Geometry: final body of the model. Coordinates: model frame, mm. A direction names the side the tool comes from. Coordinates: 2 decimals unless noted, no trailing zeros. Write each loop counter-clockwise with the first axis right and the second up, starting at its lowest first coordinate (ties: lowest second). Pieces come first, ordered by that corner, then holes.
from build123d import *

# Parameters (mm, degrees)
SKETCH_1_R      = 1.5
EXTRUDE_1_DEPTH = 6
SKETCH_2_W      = 106
SKETCH_2_H      = 60
EXTRUDE_2_DEPTH = 46


with BuildPart() as part:
    # 草图1 → 凸台-拉伸1 (new body)
    with BuildSketch(Plane(origin=(0, 0, 0), x_dir=(1, 0, 0), z_dir=(0, 1, 0))):
        Polygon((44.601753779, -30), (-44.601753779, -30), (-51.423054046, -39.075905643), (-60.615391847, -35.138784137), (-55.25, -28), (-55.25, -20), (-63.25, -20), (-63.25, 20), (-55.25, 20), (-55.25, 28), (-60.615391847, 35.138784137), (-51.423054046, 39.075905643), (-44.601753779, 30), (44.601753779, 30), (51.423054046, 39.075905643), (60.615391847, 35.138784137), (55.25, 28), (55.25, 20), (63.25, 20), (63.25, -20), (55.25, -20), (55.25, -28), (60.615391847, -35.138784137), (51.423054046, -39.075905643), align=None)
        with Locations(Location((58.25, 15, 0), (0, 0, 270))):
            Circle(SKETCH_1_R, mode=Mode.SUBTRACT)
        with Locations(Location((-58.25, 15, 0), (0, 0, 270))):
            Circle(SKETCH_1_R, mode=Mode.SUBTRACT)
        with Locations(Location((58.25, 9, 0), (0, 0, 270))):
            Circle(SKETCH_1_R, mode=Mode.SUBTRACT)
        with Locations(Location((-58.25, 9, 0), (0, 0, 270))):
            Circle(SKETCH_1_R, mode=Mode.SUBTRACT)
        with Locations(Location((58.25, -9, 0), (0, 0, 90))):
            Circle(SKETCH_1_R, mode=Mode.SUBTRACT)
        with Locations(Location((58.25, -15, 0), (0, 0, 90))):
            Circle(SKETCH_1_R, mode=Mode.SUBTRACT)
        with Locations(Location((-58.25, -9, 0), (0, 0, 90))):
            Circle(SKETCH_1_R, mode=Mode.SUBTRACT)
        with Locations(Location((-58.25, -15, 0), (0, 0, 90))):
            Circle(SKETCH_1_R, mode=Mode.SUBTRACT)
    extrude(amount=EXTRUDE_1_DEPTH)

    # 草图2 → 凸台-拉伸2 (add)
    with BuildSketch(Plane(origin=(0, 6, 0), x_dir=(1, 0, 0), z_dir=(0, 1, 0))):
        Rectangle(SKETCH_2_W, SKETCH_2_H)
    extrude(amount=EXTRUDE_2_DEPTH)


solid = part.part
Item 1: Set-up query: faces 1 (the cylindrical face through (-57.24, 2.96, -16.11)), 2 (the flat face through (-57.97, 2.96, 31.62)), 3 (the flat face through (47.96, 2.96, -34.47)), 4 (the flat face through (53, 29, 0)). Return all of +Z, -Z, +X, -X, +Y, -Y with unobstructed straight access to the full face (end or side cutting, diameter ignored); none if empty.
Derived:
face 1: +Y, -Y
face 2: -X, +Y, -Y
face 3: -Z, +Y, -Y
face 4: +Z, -Z, +X, +Y
Item 2: Section D-D, the plane y = 9.5. Output: boundary loops of the cut face in (x, z), plus the area to 3 significant figures.
Derived:
outline: (-53, -30) - (53, -30) - (53, 30) - (-53, 30) - close
area: 6,360 mm2
Item 3: Section B-B, the plane z = -9. Output: boundary loops of the cut face in (x, y), plus the area to 3 significant figures.
Derived:
outline: (-63.25, 0) - (-59.75, 0) - (-59.75, 6) - (-63.25, 6) - close; (-56.75, 0) - (56.75, 0) - (56.75, 6) - (53, 6) - (53, 52) - (-53, 52) - (-53, 6) - (-56.75, 6) - close; (59.75, 0) - (63.25, 0) - (63.25, 6) - (59.75, 6) - close
area: 5,600 mm2
Item 4: Section C-C, the plane z = 21.5. Output: boundary loops of the cut face in (x, y), plus the area to 3 significant figures.
Derived:
outline: (-55.25, 0) - (55.25, 0) - (55.25, 6) - (53, 6) - (53, 52) - (-53, 52) - (-53, 6) - (-55.25, 6) - close
area: 5,540 mm2
Item 5: Pull-direction query (Z, two-part tool) for faces 5 (the flat face through (-55.25, 3, -24)), 6 (the cylindrical face through (-59.737, 2.958, 9.195)), 7 (the flat face through (-47.96, 2.96, 34.47)), 8 (the flat face through (56, 6, -1)); classes: released by +Z, released by -Z, zero draft, split by the parting line, or undercut.
Derived:
face 5: undercut
face 6: undercut
face 7: released by +Z
face 8: zero draft
Item 6: Section A-A, the plane x = 58.25. Output: boundary loops of the cut face in (y, z), plus the area to 3 significant figures.
Derived:
outline: (0, -36.15) - (6, -36.15) - (6, -31.99) - (0, -31.99) - close; (0, -20) - (6, -20) - (6, -16.5) - (0, -16.5) - close; (0, -13.5) - (6, -13.5) - (6, -10.5) - (0, -10.5) - close; (0, -7.5) - (6, -7.5) - (6, 7.5) - (0, 7.5) - close; (0, 10.5) - (6, 10.5) - (6, 13.5) - (0, 13.5) - close; (0, 16.5) - (6, 16.5) - (6, 20) - (0, 20) - close; (0, 31.99) - (6, 31.99) - (6, 36.15) - (0, 36.15) - close
area: 218 mm2
Item 7: Pin query (flat end, axial travel): pin 1 (5 mm diameter, centred on x = -58.25, z = -9, fed in from +Y); pin 2 (6.5 mm diameter, centred on y = 2.5, z = -22.5, fed in from -X); pin 3 (3 mm diameter, centred on x = -61, y = 2, fed in from -Z); pin 4 (6 mm diameter, centred on x = 13, y = 45.5, fed in from -Z). Return the tip coordinate at first contact, or that it passes through.
Derived:
pin 1: stops at y = 6
pin 2: stops at x = -63.25
pin 3: stops at z = -35.62
pin 4: stops at z = -30
Item 8: Material intervals for probe 1 along X at (y, z) = (4, 9); probe 2 along Z at (x, y) = (52.5, 39.5); probe 3 along X at (y, z) = (25, -6.5), sorted ascending.
Derived:
probe 1: x = -63.25 to -59.75, -56.75 to 56.75, 59.75 to 63.25
probe 2: z = -30 to 30
probe 3: x = -53 to 53
